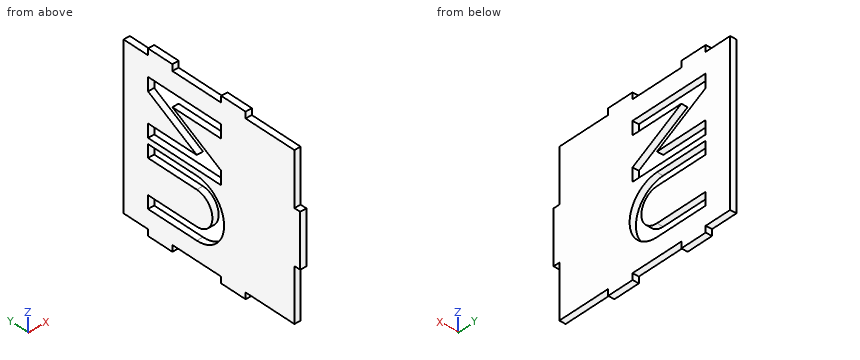
from build123d import *

# Parameters (mm, degrees)
BOSS_EXTRUDE1_DEPTH = 3


with BuildPart() as part:
    # Sketch1 → Boss-Extrude1 (new body)
    with BuildSketch(Plane(origin=(0, 0, 0), x_dir=(0, 0, -1), z_dir=(1, 0, 0))):
        Polygon((-38.1, -17.2847), (-38.1, -20.8153), (-38.1, -31.75), (-12.7, -31.75), (-12.7, -34.75), (12.7, -34.75), (12.7, -31.75), (38.1, -31.75), (38.1, -20.8153), (38.1, -17.2847), (38.1, -6.35), (41.1, -6.35), (41.1, 6.35), (38.1, 6.35), (38.1, 31.75), (41.1, 31.75), (41.1, 44.45), (38.1, 44.45), (38.1, 57.15), (-38.1, 57.15), (-38.1, 44.45), (-41.1, 44.45), (-41.1, 31.75), (-38.1, 31.75), (-38.1, 6.35), (-41.1, 6.35), (-41.1, -6.35), (-38.1, -6.35), align=None)
        Polygon((-22.288981843, 44.45), (-8.242290985, 19.05), (-8.242290985, 44.45), (-1.892290985, 44.45), (-1.892290985, 6.35), (-8.242290985, 6.35), (-22.288981843, 31.75), (-22.288981843, 6.35), (-28.638981843, 6.35), (-28.638981843, 44.45), align=None, mode=Mode.SUBTRACT)
        with BuildLine():
            Line((23.165757053, 44.45), (29.261757053, 44.45))
            Line((29.261757053, 44.45), (29.261757053, 19.05))
            ThreePointArc((29.261757053, 19.05), (15.037757053, 4.826), (0.813757053, 19.05))
            Line((0.813757053, 19.05), (0.813757053, 44.45))
            Line((0.813757053, 44.45), (6.909757053, 44.45))
            Line((6.909757053, 44.45), (6.909757053, 19.05))
            ThreePointArc((6.909757053, 19.05), (15.037757053, 10.922), (23.165757053, 19.05))
            Line((23.165757053, 19.05), (23.165757053, 44.45))
        make_face(mode=Mode.SUBTRACT)
    extrude(amount=BOSS_EXTRUDE1_DEPTH)


solid = part.part
Here's how the part is built. I have some questions about the finished solid (model axes, mm). Coordinates: 2 decimals unless noted, no trailing zeros. Order: outer loops, then holes, each group sorted by start corner. A loop starts at its lowest first (then second) coordinate and runs counter-clockwise, first axis right, second up.
Item 1: If we section it at B-B on y = 40.5: List the corners of the cut face in (x, z) for me.
Result sheet:
outline: (0, -41.1) - (3, -41.1) - (3, -29.26) - (0, -29.26) - close; (0, -23.17) - (3, -23.17) - (3, -6.91) - (0, -6.91) - close; (0, -0.81) - (3, -0.81) - (3, 1.89) - (0, 1.89) - close; (0, 8.24) - (3, 8.24) - (3, 20.1) - (0, 20.1) - close; (0, 28.64) - (3, 28.64) - (3, 41.1) - (0, 41.1) - close
Item 2: If we section it at D-D on z = -31: List the corners of the cut face in (x, y) for me, plus the area to 3 significant figures.
Result sheet:
outline: (0, -31.75) - (3, -31.75) - (3, 57.15) - (0, 57.15) - close
area: 267 mm2
Item 3: If we section it at A-A on z = -20: List the corners of the cut face in (x, y) for me.
Result sheet:
outline: (0, -31.75) - (3, -31.75) - (3, 5.72) - (0, 5.72) - close; (0, 12.61) - (3, 12.61) - (3, 57.15) - (0, 57.15) - close
Item 4: I need wall thicknesses on line 1 (Y direction, x = 2.8, z = -15); line 2 (Z direction, x = 0.4, y = 35); line 3 (Y direction, x = 2.4, z = 7). Which ranges of each line are inside material? Lowest first, please.
Result sheet:
line 1: y = -31.75 to 4.83, 10.92 to 57.15
line 2: z = -41.1 to -29.26, -23.17 to -6.91, -0.81 to 1.89, 8.24 to 17.06, 28.64 to 41.1
line 3: y = -34.75 to 6.35, 44.45 to 57.15
Item 5: If we section it at C-C on x = 2.5: State how many separate pieces and enclosed holes the cut face has, plus the area to 3 significant figures.
Result sheet:
separate pieces: 1
enclosed holes: 2
area: 5,820 mm2
Item 6: For P1, Ø1.5, axis at x = 1.5, y = 22.5, coming from the +Z side; P2, Ø4, axis at y = -13, z = 26, coming from the -X side; P3, Ø1.5, axis at x = 2, y = 30, coming from the -Z side, each with a flat end and sliding along its axis, tell me the tip position at first contact or that it passes through.
Result sheet:
P1: stops at z = 38.1
P2: stops at x = 0
P3: stops at z = -38.1
